Can you work these out from the drawing? Everything is in mm from the part's minimum corner. A direction names the side the tool comes from. Coordinates: 2 decimals unless noted, no trailing zeros. Order: outer loops, then holes, each group sorted by start corner. A loop starts at its lowest first (then second) coordinate and runs counter-clockwise, first axis right, second up. Notation, with made-up numbers: (44, 45) - (78, 45) arc R27 cw to (78, 78) - close; hole circle Ø8 at (-2, 10.5). An arc over 180 degrees is marked (long way). Use a Markdown table: item, result. Add a question column.
(1) I want a section at B-B (y = 59). List the corners of the cut face in (x, z) for me, and give its area (3 significant figures).
(2) I want a section at C-C (x = 111). List the corners of the cut face in (y, z) for me.
(3) We'd pull the mould along Z, two halves only. Please class the marked faces 1, 2 and 3: pulls with the +Z half, pulls with the -Z half, needs draft (parallel to the pull), parting line crosses it, or undercut.
(4) On a 3-axis mill with a long thin cutter (end or side, diameter ignored), from which of +Z, -Z, +X, -X, +Y, -Y can I reach the whole of each face in a straight line? I mean the marked faces 4, 5, 6 and 7. Say none if no direction works.
(5) I want a section at D-D (y = 88.5). List the corners of the cut face in (x, z) for me.
(6) I want a section at A-A (z = 40). List the corners of the cut face in (x, y) for me, and give its area (3 significant figures).
(7) If I drill on L1, parallel to X at y = 58.5, z = 24; L2, parallel to Y at x = 114.5, z = 40; L3, parallel to X at y = 100.25, z = 40, over which ranges is the centre line in solid material (lowest first)? Write a range as [from, to].
(8) For pin 1 Ø3 at (x, y) = (45, 98.5) entering from -Z, with a flat end and sliding along its axis, tell me the tip position at first contact or that it passes through.
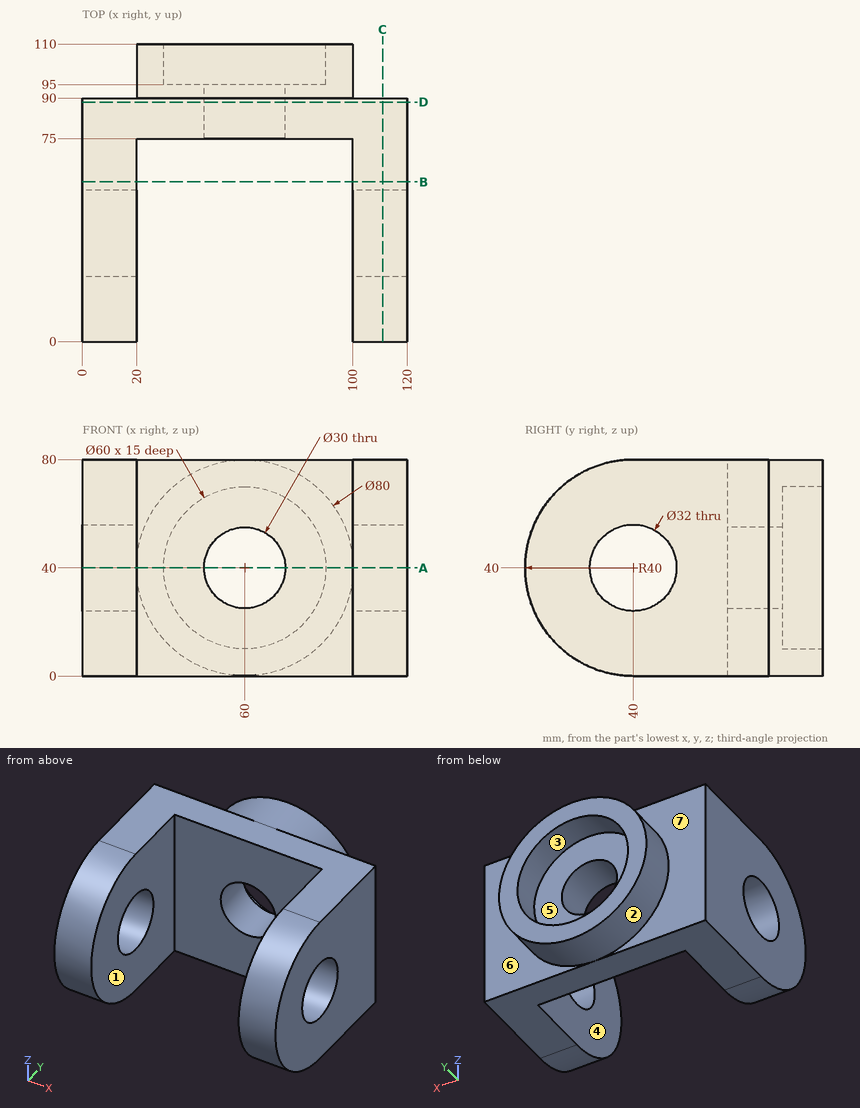
Answers follow:
| question | item | result |
|---|---|---|
| 1 | outline | (0, 0) - (20, 0) - (20, 80) - (0, 80) - close; (100, 0) - (120, 0) - (120, 80) - (100, 80) - close |
| 1 | area | 3,200 mm² |
| 2 | outline | (40, 0) - (90, 0) - (90, 80) - (40, 80) arc R40 ccw to start; hole circle Ø32 at (40, 40) |
| 3 | face 1 | needs draft |
| 3 | face 2 | parting line crosses it |
| 3 | face 3 | undercut |
| 4 | face 4 | +Z, -Z, -Y |
| 4 | face 5 | +Y |
| 4 | face 6 | +X, +Y |
| 4 | face 7 | -X, +Y |
| 5 | outline | (0, 0) - (120, 0) - (120, 80) - (0, 80) - close; hole circle Ø30 at (60, 40) |
| 6 | outline | (0, 0) - (20, 0) - (20, 24) - (0, 24) - close; (0, 56) - (20, 56) - (20, 75) - (45, 75) - (45, 95) - (30, 95) - (30, 110) - (20, 110) - (20, 90) - (0, 90) - close; (75, 75) - (100, 75) - (100, 56) - (120, 56) - (120, 90) - (100, 90) - (100, 110) - (90, 110) - (90, 95) - (75, 95) - close; (100, 0) - (120, 0) - (120, 24) - (100, 24) - close |
| 6 | area | 3,620 mm² |
| 7 | L1 | x = [0, 20], [100, 120] |
| 7 | L2 | y = [0, 24], [56, 90] |
| 7 | L3 | x = [20, 30], [90, 100] |
| 8 | pin 1 | stops at z = 2.35 |
